Read the model definition and answer for the solid it produces. Units are mm, in the model's axes. A direction names the side the tool comes from. Give positions to 0.01 mm unless a question says otherwise; leave off trailing zeros. Order: outer loops, then holes, each group sorted by start corner. A loop starts at its lowest first (then second) coordinate and runs counter-clockwise, first axis right, second up. Notation, with made-up numbers: M 37.25,82.5 L 79.25,82.5 A18 cw 79.25,113.5 Z; hole C 79,-7 d9. An arc over 180 degrees is marked long. One line per item, written item: value.
from build123d import *

# Parameters (mm, degrees)
SKETCH1_W           = 50
SKETCH1_H           = 40
BOSS_EXTRUDE1_DEPTH = 10
SKETCH3_W           = 11
SKETCH3_H           = 40
BOSS_EXTRUDE2_DEPTH = 20
SKETCH4_W           = 25
SKETCH4_H           = 10
CUT_EXTRUDE1_DEPTH  = 51
SKETCH5_R           = 2.5
CUT_EXTRUDE2_DEPTH  = 13


with BuildPart() as part:
    # Sketch1 → Boss-Extrude1 (new body)
    with BuildSketch(Plane(origin=(0, 0, 0), x_dir=(1, 0, 0), z_dir=(0, 1, 0))):
        with Locations((25, 20)):
            Rectangle(SKETCH1_W, SKETCH1_H)
    extrude(amount=BOSS_EXTRUDE1_DEPTH)

    # Sketch3 → Boss-Extrude2 (add)
    with BuildSketch(Plane(origin=(0, 10, 0), x_dir=(1, 0, 0), z_dir=(0, 1, 0))):
        with Locations((5.5, 20)):
            Rectangle(SKETCH3_W, SKETCH3_H)
    boss_extrude2 = extrude(amount=BOSS_EXTRUDE2_DEPTH)

    # Mirror1: Boss-Extrude2 across plane
    add(boss_extrude2.mirror(Plane.ZY.offset(-25)))

    # Sketch4 → Cut-Extrude1 (cut, through all)
    with BuildSketch(Plane(origin=(50, 0, 0), x_dir=(0, 0, -1), z_dir=(1, 0, 0))):
        with Locations((20, 22)):
            Rectangle(SKETCH4_W, SKETCH4_H)
    extrude(amount=-CUT_EXTRUDE1_DEPTH, mode=Mode.SUBTRACT)

    # Sketch5 → Cut-Extrude2 (cut)
    with BuildSketch(Plane(origin=(0, 30, 0), x_dir=(1, 0, 0), z_dir=(0, 1, 0))):
        with Locations((7.5, 20)):
            Circle(SKETCH5_R)
    cut_extrude2 = extrude(amount=-CUT_EXTRUDE2_DEPTH, mode=Mode.SUBTRACT)

    # Mirror2: Cut-Extrude2 across plane
    add(cut_extrude2.mirror(Plane.ZY.offset(-25)), mode=Mode.SUBTRACT)


solid = part.part
1) Consider probe 1 along X at (y, z) = (29.1, -20); probe 2 along Y at (x, z) = (40.5, -9.5); probe 3 along Z at (x, y) = (42.5, 28.7). Determine where each line is inside the solid, lowest interval first.
Reported:
probe 1: x = 0 to 5, 10 to 11, 39 to 40, 45 to 50
probe 2: y = 0 to 17, 27 to 30
probe 3: z = -40 to -22.5, -17.5 to 0
2) Find section B-B, the plane z = -8.5. Write down the section's boundary in (x, y).
Reported:
outline: M 0,0 L 50,0 L 50,17 L 39,17 L 39,10 L 11,10 L 11,17 L 0,17 Z; M 0,27 L 11,27 L 11,30 L 0,30 Z; M 39,27 L 50,27 L 50,30 L 39,30 Z
3) Determine the mould class of faces 1 (the face through (9, 29, -22)), 2 (the face through (45, 17, -20)), 3 (the face through (25, 10, -20)) for opening direction Y: +Y half, -Y half, draft (parallel to the pull), parting line (faces both ways), or undercut.
Reported:
face 1: draft
face 2: undercut
face 3: +Y half
4) Find section C-C, the plane x = 7.5. Write down the section's boundary in (y, z), plus the area to 3 significant figures.
Reported:
outline: M 0,-40 L 30,-40 L 30,-22.5 L 27,-22.5 L 27,-32.5 L 17,-32.5 L 17,-7.5 L 27,-7.5 L 27,-17.5 L 30,-17.5 L 30,0 L 0,0 Z
area: 935 mm^2
5) Which of the six approach directions +Z, -Z, +X, -X, +Y, -Y give full straight-line access (tool end or side, diameter ignored) to faces 4 (the face through (25, 8, 0)), 5 (the face through (11, 15, -20)), 6 (the face through (41, 29, -22)), 7 (the face through (46, 27, -20))?
Reported:
face 4: +Z, +X, -X, +Y, -Y
face 5: +Z, -Z, +Y
face 6: +Y
face 7: +X, -X
6) Find section D-D, the plane x = 43. Write down the section's boundary in (y, z).
Reported:
outline: M 0,-40 L 30,-40 L 30,-22.45 L 27,-22.45 L 27,-32.5 L 17,-32.5 L 17,-7.5 L 27,-7.5 L 27,-17.55 L 30,-17.55 L 30,0 L 0,0 Z
7) This flat-tipped pin is pushed along its axis until it touches: pin 1 Ø8.5 at (x, z) = (19, -26) entering from +Y. Where does it stop, or does it pass through?
Reported:
pin 1: stops at y = 10
8) Find section A-A, the plane z = -20. Write down the section's boundary in (x, y).
Reported:
outline: M 0,0 L 50,0 L 50,17 L 39,17 L 39,10 L 11,10 L 11,17 L 0,17 Z; M 0,27 L 5,27 L 5,30 L 0,30 Z; M 10,27 L 11,27 L 11,30 L 10,30 Z; M 39,27 L 40,27 L 40,30 L 39,30 Z; M 45,27 L 50,27 L 50,30 L 45,30 Z
